```python
from build123d import *

# Parameters (mm, degrees)
SKETCH_W        = 130
SKETCH_H        = 68
PAD_DEPTH       = 70
SKETCH001_W     = 122
SKETCH001_H     = 64
POCKET_DEPTH    = 62
SKETCH002_W     = 126
SKETCH002_H     = 3
POCKET001_DEPTH = 68.001
SKETCH004_R     = 1.5
POCKET002_DEPTH = 5
SKETCH005_R     = 8.5
POCKET003_DEPTH = 70.001


with BuildPart() as part:
    # Sketch (on XY_Plane of Origin) → Pad (new body)
    with BuildSketch(Plane.XY):
        with Locations((15.008508, 3.133008)):
            Rectangle(SKETCH_W, SKETCH_H)
    extrude(amount=PAD_DEPTH)

    # Sketch001 (on Face6 of Pad) → Pocket (cut)
    with BuildSketch(Plane.XY.offset(70)):
        with Locations((15.008508, 3.133008)):
            Rectangle(SKETCH001_W, SKETCH001_H)
    extrude(amount=-POCKET_DEPTH, mode=Mode.SUBTRACT)

    # Sketch002 (on Face3 of Pocket) → Pocket001 (cut, through all)
    with BuildSketch(Plane.XZ.offset(30.866992)):
        with Locations((15.643498, 64.782843)):
            Rectangle(SKETCH002_W, SKETCH002_H)
    extrude(amount=-POCKET001_DEPTH, mode=Mode.SUBTRACT)

    # Sketch004 (on Face6 of Pocket001) → Pocket002 (cut)
    with BuildSketch(Plane.YZ.offset(80.008508)):
        with Locations((-18.646347, 35.954605)):
            Circle(SKETCH004_R)
        with Locations((-13.646347, 35.954605)):
            Circle(SKETCH004_R)
        with Locations((-8.646347, 35.954605)):
            Circle(SKETCH004_R)
        with Locations((-18.687416, 30.954774)):
            Circle(SKETCH004_R)
        with Locations((-13.687416, 30.954774)):
            Circle(SKETCH004_R)
        with Locations((-8.687416, 30.954774)):
            Circle(SKETCH004_R)
        with Locations((-18.728485, 25.954942)):
            Circle(SKETCH004_R)
        with Locations((-13.728485, 25.954942)):
            Circle(SKETCH004_R)
        with Locations((-8.728485, 25.954942)):
            Circle(SKETCH004_R)
        with Locations((-18.646347, 20.885028)):
            Circle(SKETCH004_R)
        with Locations((-13.646347, 20.885028)):
            Circle(SKETCH004_R)
        with Locations((-8.646347, 20.885028)):
            Circle(SKETCH004_R)
        with Locations((-18.687416, 15.885197)):
            Circle(SKETCH004_R)
        with Locations((-13.687416, 15.885197)):
            Circle(SKETCH004_R)
        with Locations((-8.687416, 15.885197)):
            Circle(SKETCH004_R)
        with Locations((-18.728485, 10.885365)):
            Circle(SKETCH004_R)
        with Locations((-13.728485, 10.885365)):
            Circle(SKETCH004_R)
        with Locations((-8.728485, 10.885365)):
            Circle(SKETCH004_R)
        with Locations((-18.22651, 50.948728)):
            Circle(SKETCH004_R)
        with Locations((-13.22651, 50.948728)):
            Circle(SKETCH004_R)
        with Locations((-8.22651, 50.948728)):
            Circle(SKETCH004_R)
        with Locations((-18.267579, 45.948897)):
            Circle(SKETCH004_R)
        with Locations((-13.267579, 45.948897)):
            Circle(SKETCH004_R)
        with Locations((-8.267579, 45.948897)):
            Circle(SKETCH004_R)
        with Locations((-18.308648, 40.949065)):
            Circle(SKETCH004_R)
        with Locations((-13.308648, 40.949065)):
            Circle(SKETCH004_R)
        with Locations((-8.308648, 40.949065)):
            Circle(SKETCH004_R)
    extrude(amount=-POCKET002_DEPTH, mode=Mode.SUBTRACT)

    # Sketch005 (on Face4 of Pocket002) → Pocket003 (cut, through all)
    with BuildSketch(Plane(origin=(0, 0, 0), x_dir=(1, 0, 0), z_dir=(0, 0, -1))):
        with Locations((39.327614, 12.574978)):
            Circle(SKETCH005_R)
        with Locations((39.327614, -14.425022)):
            Circle(SKETCH005_R)
    extrude(amount=-POCKET003_DEPTH, mode=Mode.SUBTRACT)


solid = part.part
```
Could you check a few things on this model? Use its own coordinates, in mm. A direction names the side the tool comes from. Round coordinates to 2 decimals unless told otherwise and drop trailing zeros. Loops run counter-clockwise (first coordinate to the right, second up) from the corner with the lowest first, then second, coordinate; pieces in that order, holes last. Notation, with made-up numbers: M -38,81.25 L -32,81.25 A17 cw -32,97.25 Z; hole C 47,5.25 d7. An arc over 180 degrees is marked long. Put each result on its own line as item: value.
Q1. For pin 1 (2.5 mm diameter, centred on y = -18.69, z = 30.95, fed in from +X); pin 2 (10 mm diameter, centred on x = -11, y = -10, fed in from +Z); pin 3 (2 mm diameter, centred on x = -4, y = 28, fed in from -Z), each with a flat end and sliding along its axis, tell me the tip position at first contact or that it passes through.
Check result:
pin 1: x = -45.99
pin 2: z = 8
pin 3: z = 0
Q2. Imagine slicing it at A-A (x = -15). Write out the boundary of the cut face in (y, z).
Check result:
outline: M -30.87,0 L 37.13,0 L 37.13,63.28 L 35.13,63.28 L 35.13,8 L -28.87,8 L -28.87,63.28 L -30.87,63.28 Z; M -30.87,66.28 L -28.87,66.28 L -28.87,70 L -30.87,70 Z; M 35.13,66.28 L 37.13,66.28 L 37.13,70 L 35.13,70 Z
Q3. I need wall thicknesses on probe 1 along X at (y, z) = (1, 40.5); probe 2 along Y at (x, z) = (56, 35.5); probe 3 along X at (y, z) = (-1, 66). Which ranges of each line are inside material? Lowest first, please.
Check result:
probe 1: -49.99 to -45.99, 76.01 to 80.01
probe 2: -30.87 to -28.87, 35.13 to 37.13
probe 3: -49.99 to -47.36, 78.64 to 80.01
Q4. Imagine slicing it at C-C (x = 43.5). Write out the boundary of the cut face in (y, z).
Check result:
outline: M -30.87,0 L -19.98,0 L -19.98,8 L -28.87,8 L -28.87,63.28 L -30.87,63.28 Z; M -30.87,66.28 L -28.87,66.28 L -28.87,70 L -30.87,70 Z; M -5.17,0 L 7.02,0 L 7.02,8 L -5.17,8 Z; M 21.83,0 L 37.13,0 L 37.13,63.28 L 35.13,63.28 L 35.13,8 L 21.83,8 Z; M 35.13,66.28 L 37.13,66.28 L 37.13,70 L 35.13,70 Z
Q5. Imagine slicing it at B-B (z = 55.5). Write out the boundary of the cut face in (x, y), then the cut area to 3 significant figures.
Check result:
outline: M -49.99,-30.87 L 80.01,-30.87 L 80.01,37.13 L -49.99,37.13 Z; hole M -45.99,-28.87 L 76.01,-28.87 L 76.01,35.13 L -45.99,35.13 Z
area: 1,030 mm2
Q6. Thinking about a two-plate mould opening in Z: for faces 1 (the face through (32.582, 19.597, 3.944)), 2 (the face through (-47.357, 3, 65)), 3 (the face through (9.9, -29.4, 70)), 4 (the face through (78.037, -11.923, 40.375)), which applies, released by +Z, released by -Z, zero draft, split by the parting line, or undercut?
Check result:
face 1: zero draft
face 2: undercut
face 3: released by +Z
face 4: undercut
Q7. Imagine slicing it at D-D (y = 26). Write out the boundary of the cut face in (x, z), then the cut area to 3 significant figures.
Check result:
outline: M -49.99,0 L 80.01,0 L 80.01,70 L 76.01,70 L 76.01,66.28 L 78.64,66.28 L 78.64,63.28 L 76.01,63.28 L 76.01,8 L -45.99,8 L -45.99,63.28 L -47.36,63.28 L -47.36,66.28 L -45.99,66.28 L -45.99,70 L -49.99,70 Z
area: 1,520 mm2
Q8. On a 3-axis mill with a long thin cutter (end or side, diameter ignored), from which of +Z, -Z, +X, -X, +Y, -Y can I reach the whole of each face in a straight line? I mean faces 5 (the face through (80.009, 3, 35)), 6 (the face through (78.037, -13.883, 17.372)), 7 (the face through (14, 35.133, 68)), 8 (the face through (34, 36, 63.283)). Say none if no direction works.
Check result:
face 5: +Z, -Z, +X, +Y, -Y
face 6: +X
face 7: +Z
face 8: +Y, -Y
